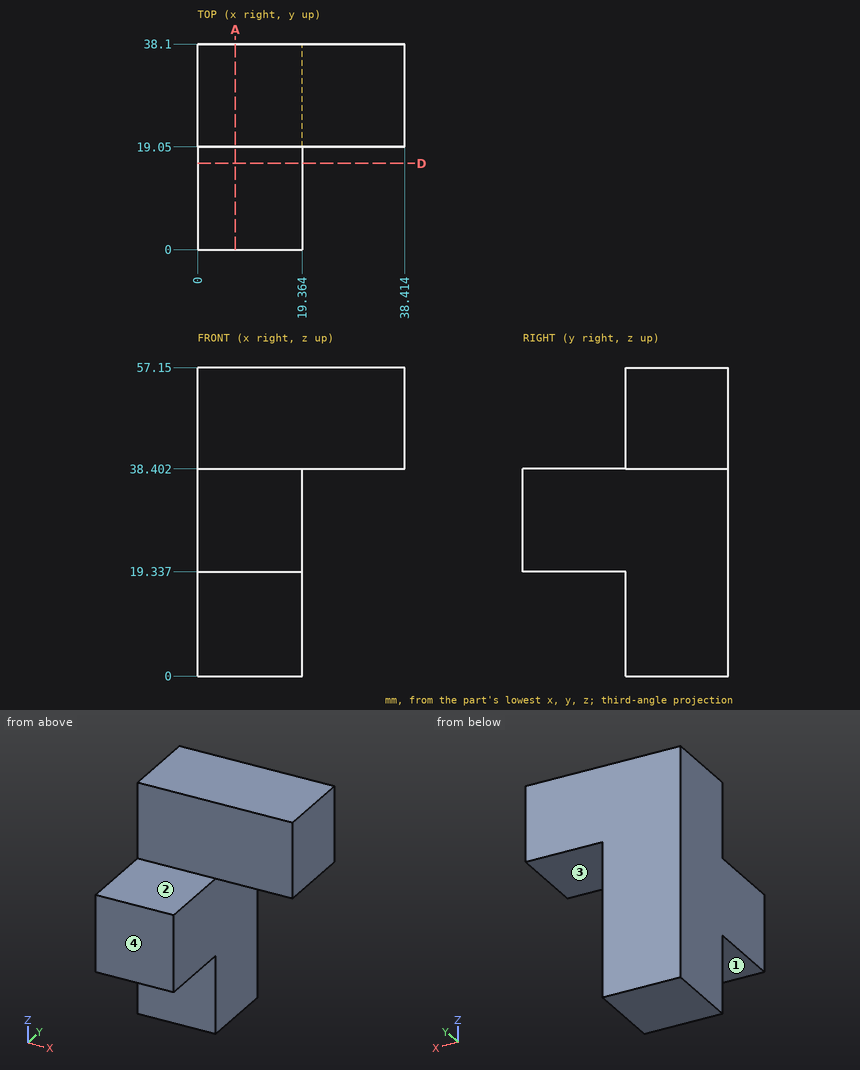
Can you work these out from the drawing? Everything is in mm from the part's minimum corner. A direction names the side the tool comes from. Round coordinates to 2 decimals unless told otherwise and drop trailing zeros. Loops run counter-clockwise (first coordinate to the right, second up) from the corner with the lowest first, then second, coordinate; pieces in that order, holes last. Notation, with made-up numbers: (44.25, 43.25) -> (65.25, 43.25) arc R24 ccw to (65.25, 67.25) -> close; hole circle Ø6 at (25.5, -9.5). An arc over 180 degrees is marked (long way). Put each result on its own line as item: value.
Q1. Please list where these lines run through material, in increasing order: line 1 (Y direction, x = 8, z = 10.5); line 2 (Z direction, x = 24.5, y = 27); line 3 (Z direction, x = 17, y = 18). Write a range as from..to.
Checks:
line 1: 19.05..38.1
line 2: 38.4..57.15
line 3: 19.34..38.4
Q2. Which directions (+Z, -Z, +X, -X, +Y, -Y) give clear straight access to the entire face, cutting with the end or side of a thin tool? Please do the marked faces 1, 2, 3 and 4.
Checks:
face 1: -Z, +X, -X, -Y
face 2: +Z, +X, -X, -Y
face 3: -Z, +X, +Y, -Y
face 4: +Z, -Z, +X, -X, -Y
Q3. I want a section at A-A on x = 7. Write out the boundary of the cut face in (y, z).
Checks:
outline: (0, 19.34) -> (19.05, 19.34) -> (19.05, 0) -> (38.1, 0) -> (38.1, 57.15) -> (19.05, 57.15) -> (19.05, 38.4) -> (0, 38.4) -> close
Q4. For pin 1 Ø21 at (x, y) = (31.5, 32) entering from -Z; pin 2 Ø9.5 at (x, z) = (10, 6.5) entering from -Y; pin 3 Ø6 at (y, z) = (6.5, 33) entering from +X; pin 4 Ø12 at (x, z) = (26, 6.5) entering from +Y, each with a flat end and sliding along its axis, tell me the tip position at first contact or that it passes through.
Checks:
pin 1: z = 38.4
pin 2: y = 19.05
pin 3: x = 19.36
pin 4: through
Q5. I want a section at D-D on y = 16. Write out the boundary of the cut face in (x, z) (1 decimal).
Checks:
outline: (0, 19.3) -> (19.4, 19.3) -> (19.4, 38.4) -> (0, 38.4) -> close
